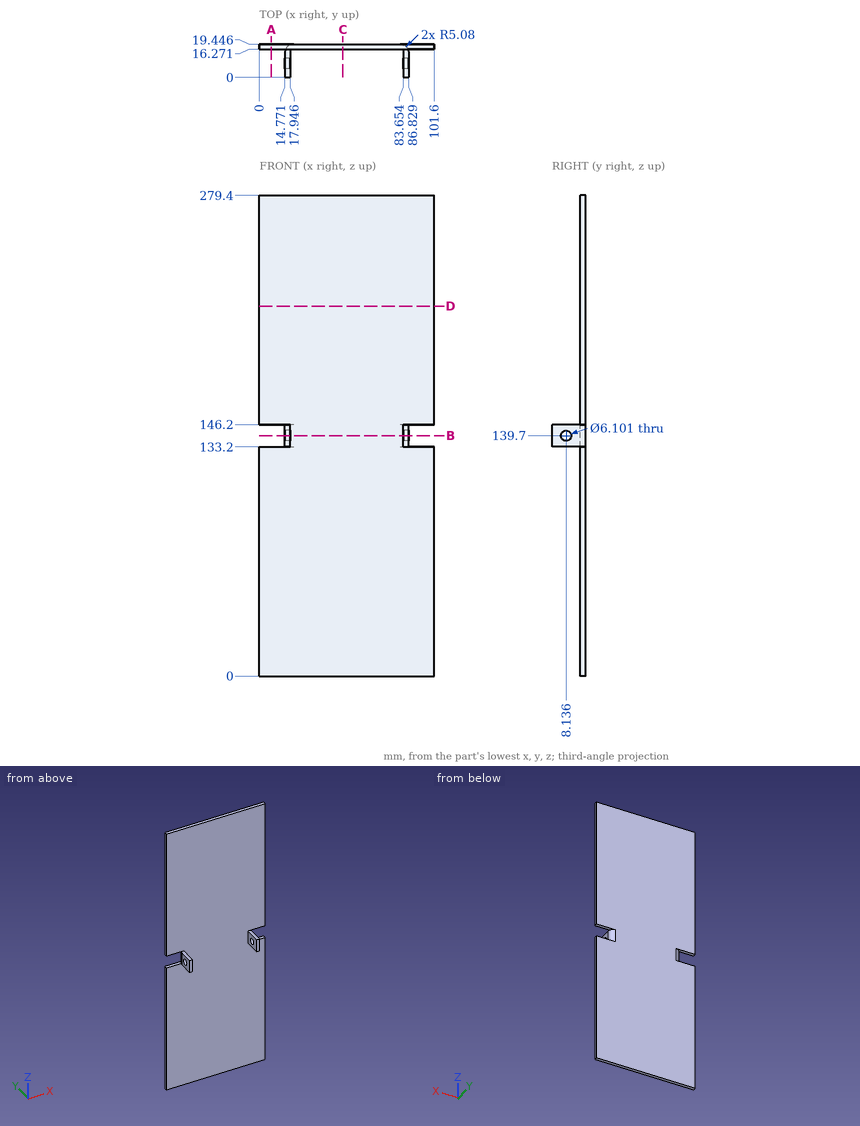
Study the drawing (mm; zero at the part's minimum x, y, z) and answer. Round coordinates to 2 decimals unless told otherwise and drop trailing zeros. Write each loop counter-clockwise with the first axis right and the second up, starting at its lowest first coordinate (ties: lowest second). Pieces come first, ordered by that corner, then holes. Notation, with made-up numbers: (6, -37) - (28, -37) arc R30 ccw to (28, -9) - close; hole circle Ø1 at (86.25, 13.5). An arc over 180 degrees is marked (long way). Use a Markdown table: item, result. Add a question column.
1. The part is cut by section D-D (z = 215). Write down the section's boundary in (x, y).
2. Consider line 1 (Y direction, x = 76, z = 85.5); line 2 (Y direction, x = 85, z = 139.7) (1 decimal); line 3 (Y direction, x = 85, z = 139) (1 decimal). Determine where each line is inside the solid, lowest interval first.
3. The part is cut by section C-C (x = 48.5). Write down the section's boundary in (y, z).
4. Flat-ended cylindrical pins translate along their axes: P1, Ø6.5, axis at y = 11.5, z = 140.5, coming from the +X side; P2, Ø10.5, axis at y = 7.5, z = 140, coming from the -X side; P3, Ø1, axis at x = 16, y = 6, coming from the -Z side. Find the tip coordinate at first contact, or state that the pin passes through.
5. The part is cut by section B-B (z = 139.7). Write down the section's boundary in (x, y) (1 decimal), and give its area (3 significant figures).
6. The part is cut by section A-A (x = 7). Write down the section's boundary in (y, z).
Reported:
| question | item | result |
|---|---|---|
| 1 | outline | (0, 16.27) - (101.6, 16.27) - (101.6, 19.45) - (0, 19.45) - close |
| 2 | line 1 | 16.27 to 19.45 |
| 2 | line 2 | 0 to 5.1, 11.2 to 18.3 |
| 2 | line 3 | 0 to 5.2, 11.1 to 18.3 |
| 3 | outline | (16.27, 0) - (19.45, 0) - (19.45, 279.4) - (16.27, 279.4) - close |
| 4 | P1 | x = 86.83 |
| 4 | P2 | x = 14.77 |
| 4 | P3 | z = 133.2 |
| 5 | outline | (14.8, 0) - (17.9, 0) - (17.9, 5.1) - (14.8, 5.1) - close; (14.8, 11.2) - (17.9, 11.2) - (17.9, 16.3) - (83.7, 16.3) - (83.7, 11.2) - (86.8, 11.2) - (86.8, 14.4) arc R5.1 ccw to (81.7, 19.4) - (19.9, 19.4) arc R5.1 ccw to (14.8, 14.4) - close; (83.7, 0) - (86.8, 0) - (86.8, 5.1) - (83.7, 5.1) - close |
| 5 | area | 282 mm^2 |
| 6 | outline | (16.27, 0) - (19.45, 0) - (19.45, 133.2) - (16.27, 133.2) - close; (16.27, 146.2) - (19.45, 146.2) - (19.45, 279.4) - (16.27, 279.4) - close |
